Geometry: final body of the model. Coordinates: model frame, mm. A direction names the side the tool comes from. Give positions to 0.01 mm unless a question says otherwise; leave off trailing zeros. Order: outer loops, then holes, each group sorted by start corner. A loop starts at its lowest first (then second) coordinate and runs counter-clockwise, first axis right, second up. Notation, with made-up numbers: M 89.25,-0.5 L 101.25,-0.5 A21 ccw 101.25,33.5 Z; hole C 67,-23 d5. An arc over 180 degrees is marked long. Use CSV: the item, a comma, the result in double quotes.
```python
from build123d import *

# Parameters (mm, degrees)
BOSS_EXTRU_1_DEPTH      = 120
ESQUISSE2_W             = 30.2
ESQUISSE2_H             = 5.2
ENL_V_MAT_EXTRU_1_DEPTH = 10
ESQUISSE3_R             = 2.05
ENL_V_MAT_EXTRU_2_DEPTH = 121.657614762
CONG_2_R                = 1.5
ESQUISSE4_R             = 2.5
ENL_V_MAT_EXTRU_3_DEPTH = 5
CONG_2_OF_SYM_TRIE6_R   = 1.5


with BuildPart() as part:
    # Esquisse1 → Boss.-Extru.1 (new body)
    with BuildSketch(Plane(origin=(0, 0, 0), x_dir=(0, 0, -1), z_dir=(1, 0, 0))):
        with BuildLine():
            Line((6, 7.5), (-6, 7.5))
            ThreePointArc((-6, 7.5), (-7.060660172, 7.060660172), (-7.5, 6))
            Line((-7.5, 6), (-7.5, -6))
            ThreePointArc((-7.5, -6), (-7.060660172, -7.060660172), (-6, -7.5))
            Line((-6, -7.5), (6, -7.5))
            ThreePointArc((6, -7.5), (7.060660172, -7.060660172), (7.5, -6))
            Line((7.5, -6), (7.5, 6))
            ThreePointArc((7.5, 6), (7.060660172, 7.060660172), (6, 7.5))
        make_face()
    boss_extru_1 = extrude(amount=BOSS_EXTRU_1_DEPTH)

    # Esquisse2 → Enlèv. mat.-Extru.1 (cut)
    with BuildSketch(Plane.XY.offset(7.5)):
        Rectangle(ESQUISSE2_W, ESQUISSE2_H)
        with Locations((75, 0)):
            Rectangle(ESQUISSE2_W, ESQUISSE2_H)
    enl_v_mat_extru_1 = extrude(amount=-ENL_V_MAT_EXTRU_1_DEPTH, mode=Mode.SUBTRACT)

    # Esquisse3 → Enlèv. mat.-Extru.2 (cut, symmetric)
    with BuildSketch(Plane(origin=(0, -2.6, 0), x_dir=(1, 0, 0), z_dir=(0, 1, 0))):
        with Locations(Location((8, -2.5, 0), (0, 0, 180))):
            Circle(ESQUISSE3_R)
        with Locations(Location((67, -2.5, 0), (0, 0, 180))):
            Circle(ESQUISSE3_R)
        with Locations((83, -2.5)):
            Circle(ESQUISSE3_R)
    enl_v_mat_extru_2 = extrude(amount=ENL_V_MAT_EXTRU_2_DEPTH, both=True, mode=Mode.SUBTRACT)

    # Congé2
    cong_2_edges = [part.edges().sort_by_distance(p)[0] for p in [
        (120, 7.060660172, 7.060660172),
        (120, 0, 7.5),
        (120, -7.060660172, 7.060660172),
        (120, -7.5, 0),
        (120, -7.060660172, -7.060660172),
        (120, 0, -7.5),
        (120, 7.060660172, -7.060660172),
        (120, 7.5, 0),
    ]]
    fillet(cong_2_edges, radius=CONG_2_R)

    # Esquisse4 → Enlèv. mat.-Extru.3 (cut)
    with BuildSketch(Plane(origin=(120, 0, 0), x_dir=(0, 0, -1), z_dir=(1, 0, 0))):
        Circle(ESQUISSE4_R)
    enl_v_mat_extru_3 = extrude(amount=-ENL_V_MAT_EXTRU_3_DEPTH, mode=Mode.SUBTRACT)

    # Symétrie6: Boss.-Extru.1, Enlèv. mat.-Extru.1, Enlèv. mat.-Extru.2, Enlèv. mat.-Extru.3 across plane
    add(boss_extru_1.mirror(Plane(origin=(0, 6, -6), x_dir=(0, 0, 1), z_dir=(-1, 0, 0))))
    add(enl_v_mat_extru_1.mirror(Plane(origin=(0, 6, -6), x_dir=(0, 0, 1), z_dir=(-1, 0, 0))), mode=Mode.SUBTRACT)
    add(enl_v_mat_extru_2.mirror(Plane(origin=(0, 6, -6), x_dir=(0, 0, 1), z_dir=(-1, 0, 0))), mode=Mode.SUBTRACT)
    add(enl_v_mat_extru_3.mirror(Plane(origin=(0, 6, -6), x_dir=(0, 0, 1), z_dir=(-1, 0, 0))), mode=Mode.SUBTRACT)

    # Congé2 of Symétrie6
    cong_2_of_sym_trie6_edges = [part.edges().sort_by_distance(p)[0] for p in [
        (-120, 7.060660172, 7.060660172),
        (-120, 0, 7.5),
        (-120, -7.060660172, 7.060660172),
        (-120, -7.5, 0),
        (-120, -7.060660172, -7.060660172),
        (-120, 0, -7.5),
        (-120, 7.060660172, -7.060660172),
        (-120, 7.5, 0),
    ]]
    fillet(cong_2_of_sym_trie6_edges, radius=CONG_2_OF_SYM_TRIE6_R)


solid = part.part
```
1. Line query: line 1 (Z direction, x = -8, y = -4.85); line 2 (Y direction, x = 64, z = 1.5); line 3 (Z direction, x = 64, y = -2.5). Output: solid intervals per line, ascending.
Answer:
line 1,"-7.5 to 0.45, 4.55 to 7.5"
line 2,"-7.5 to -2.6, 2.6 to 7.5"
line 3,"-7.5 to -2.5"
2. Section B-B, the plane y = 0. Return the cut outline in (x, z).
Answer:
outline,"M -120,-6 A1.5 ccw -118.5,-7.5 L 118.5,-7.5 A1.5 ccw 120,-6 L 120,-2.5 L 115,-2.5 L 115,2.5 L 120,2.5 L 120,6 A1.5 ccw 118.5,7.5 L 90.1,7.5 L 90.1,-2.5 L 59.9,-2.5 L 59.9,7.5 L 15.1,7.5 L 15.1,-2.5 L -15.1,-2.5 L -15.1,7.5 L -59.9,7.5 L -59.9,-2.5 L -90.1,-2.5 L -90.1,7.5 L -118.5,7.5 A1.5 ccw -120,6 L -120,2.5 L -115,2.5 L -115,-2.5 L -120,-2.5 Z"
3. Pull-direction query (Y, two-part tool) for faces 1 (the face through (0, 2.6, 3)), 2 (the face through (2, 7.5, 0)), 3 (the face through (-10.05, 5.02, 2.59)); classes: +Y half, -Y half, draft (parallel to the pull), parting line (faces both ways), or undercut.
Answer:
face 1,"undercut"
face 2,"+Y half"
face 3,"draft"
4. Pin query (flat end, axial travel): pin 1 Ø3.5 at (x, z) = (-67, 2.5) entering from -Y (3 decimals); pin 2 Ø2.5 at (y, z) = (0.5, -1) entering from -X. Return the tip coordinate at first contact, or that it passes through.
Answer:
pin 1,"through"
pin 2,"x = -115"
5. Reachability of faces 4 (the face through (115, 0, 0)), 5 (the face through (-115, 0, 0)), 6 (the face through (-75, 0, -2.5)) from +Z, -Z, +X, -X, +Y, -Y: full face, straight path, thin tool, end or side. Return the list, or none.
Answer:
face 4,"+X"
face 5,"-X"
face 6,"+Z"
6. Section A-A, the plane x = 8. Return the cut outline in (y, z), plus the area to 3 significant figures.
Answer:
outline,"M -7.5,-6 A1.5 ccw -6,-7.5 L 6,-7.5 A1.5 ccw 7.5,-6 L 7.5,0.45 L 2.6,0.45 L 2.6,-2.5 L -2.6,-2.5 L -2.6,0.45 L -7.5,0.45 Z; M -7.5,4.55 L -2.6,4.55 L -2.6,7.5 L -6,7.5 A1.5 ccw -7.5,6 Z; M 2.6,4.55 L 7.5,4.55 L 7.5,6 A1.5 ccw 6,7.5 L 2.6,7.5 Z"
area,"131 mm2"
